Part print with two shaded views. Sizes in mm from the minimum x, y, z corner. Coordinates: 2 decimals unless noted, no trailing zeros. Answer in a Markdown table with one row per item. Add a question column.
Q1. Band-saw the part on A-A (z = 8.75). State how many separate pieces and enclosed holes the cut face has.
Q2. Drill centre lines: line 1 along Y through (x, z) = (2.25, 7.5) (1 decimal); line 2 along Y through (x, z) = (0.75, 11.75) (1 decimal); line 3 along Y through (x, z) = (5.5, 7) (1 decimal). Where is each one in solid material? Low to high. Write a range as from..to.
Q3. Two-plate mould, pull along Z, no slides. Class the marked faces 1, 2 and 3: +Z half, -Z half, draft (parallel to the pull), parting line (faces both ways), or undercut.
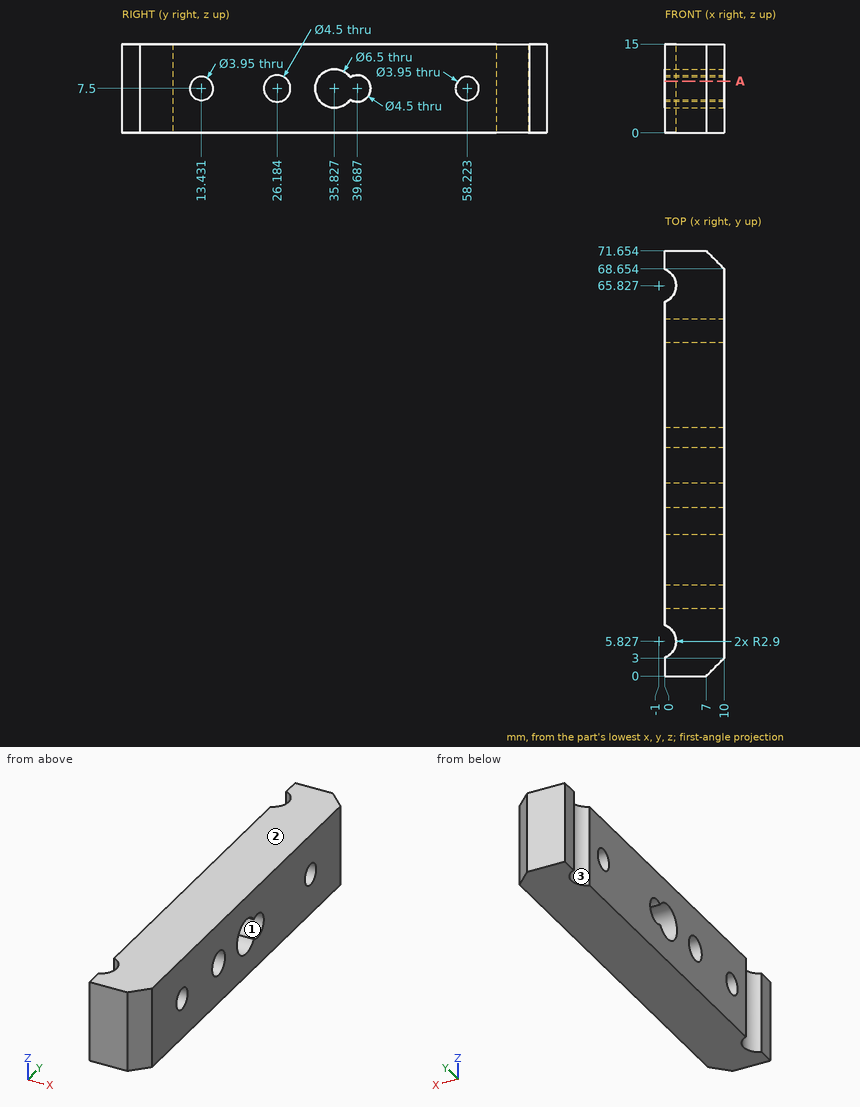
Checked values:
| question | item | result |
|---|---|---|
| 1 | separate pieces | 5 |
| 1 | enclosed holes | 0 |
| 2 | line 1 | y = 0..11.5, 15.4..23.9, 28.4..32.6, 41.9..56.2, 60.2..71.7 |
| 2 | line 2 | y = 0..3.5, 8.1..63.5, 68.1..71.7 |
| 2 | line 3 | y = 0..11.5, 15.3..24, 28.4..32.6, 41.9..56.3, 60.1..71.7 |
| 3 | face 1 | undercut |
| 3 | face 2 | +Z half |
| 3 | face 3 | draft |
